Here's how the part is built. I have some questions about the finished solid (model axes, mm). Round coordinates to 2 decimals unless told otherwise and drop trailing zeros. Write each loop counter-clockwise with the first axis right and the second up, starting at its lowest first coordinate (ties: lowest second). Pieces come first, ordered by that corner, then holes. Notation, with made-up numbers: (-4, -22) -> (13, -22) arc R25 cw to (13, 8) -> close; hole circle Ø10 at (-28.75, 33.25). An arc over 180 degrees is marked (long way). Answer as CSV lines item,"result".
from build123d import *

# Parameters (mm, degrees)
F0_W     = 60
F0_H     = 30
F1_DEPTH = 90
F3_R     = 1.25
F4_DEPTH = 40
F5_R     = 1.25
F6_DEPTH = 40


with BuildPart() as f1:
    # F0 (on Top) → F1 (new body)
    with BuildSketch(Plane.XY):
        Rectangle(F0_W, F0_H)
    extrude(amount=F1_DEPTH)

    # F3 (on face) → F4 (cut)
    with BuildSketch(Plane(origin=(0, 0, 0), x_dir=(1, 0, 0), z_dir=(0, 0, -1))):
        with Locations((-15, 0)):
            Circle(F3_R)
        with Locations((15, 0)):
            Circle(F3_R)
    extrude(amount=-F4_DEPTH, mode=Mode.SUBTRACT)

    # F5 (on face) → F6 (cut)
    with BuildSketch(Plane.XY.offset(90)):
        with Locations((-15, 0)):
            Circle(F5_R)
        with Locations((15, 0)):
            Circle(F5_R)
    extrude(amount=-F6_DEPTH, mode=Mode.SUBTRACT)


solid = f1.part
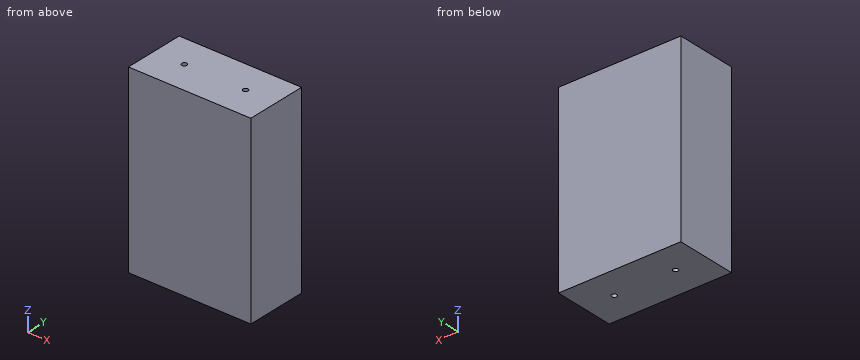
Item 1: Will this pin go through, and if not, where does the flat tip stop? pin 1 (1.5 mm diameter, centred on x = -15, y = 0, fed in from +Z).
Results found:
pin 1,"stops at z = 50"
Item 2: Suppose I cut it at A-A, the plane y = 0. List the corners of the cut face in (x, z) for me.
Results found:
outline,"(-30, 0) -> (-16.25, 0) -> (-16.25, 40) -> (-13.75, 40) -> (-13.75, 0) -> (13.75, 0) -> (13.75, 40) -> (16.25, 40) -> (16.25, 0) -> (30, 0) -> (30, 90) -> (16.25, 90) -> (16.25, 50) -> (13.75, 50) -> (13.75, 90) -> (-13.75, 90) -> (-13.75, 50) -> (-16.25, 50) -> (-16.25, 90) -> (-30, 90) -> close"
Item 3: I need wall thicknesses on L1, parallel to X at y = 0, z = 29.5; L2, parallel to Y at x = 15, z = 74; L3, parallel to X at y = 0.75, z = 26.5. Which ranges of each line are inside material? Lowest first, please.
Results found:
L1,"x = -30 to -16.25, -13.75 to 13.75, 16.25 to 30"
L2,"y = -15 to -1.25, 1.25 to 15"
L3,"x = -30 to -16, -14 to 14, 16 to 30"
Item 4: Suppose I cut it at B-B, the plane x = -15. List the corners of the cut face in (y, z) for me.
Results found:
outline,"(-15, 0) -> (-1.25, 0) -> (-1.25, 40) -> (1.25, 40) -> (1.25, 0) -> (15, 0) -> (15, 90) -> (1.25, 90) -> (1.25, 50) -> (-1.25, 50) -> (-1.25, 90) -> (-15, 90) -> close"
